Input: part model. Units: mm. Frame: model coordinates. Round coordinates to 2 decimals unless told otherwise and drop trailing zeros. Order: outer loops, then holes, each group sorted by start corner. A loop starts at its lowest first (then second) coordinate and runs counter-clockwise, first axis right, second up. Notation, with made-up numbers: (65, 25) - (84, 25) arc R18 cw to (84, 40) - close; hole circle Ø4 at (-6, -5.75). An arc over 180 degrees is marked (long way). One line per item, written item: value. Start each with the question number.
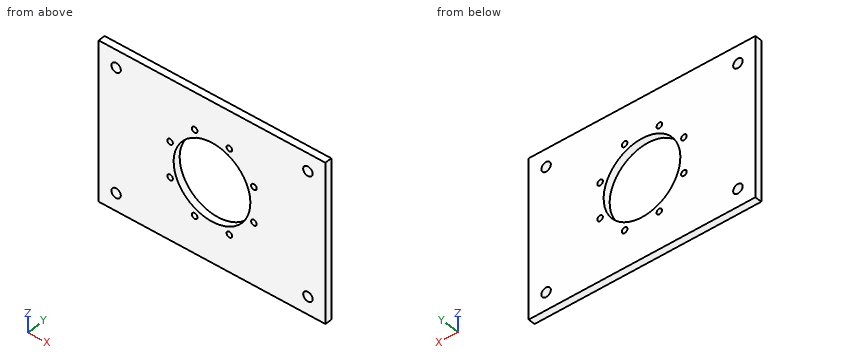
from build123d import *

# Parameters (mm, degrees)
SKETCH1_W           = 325
SKETCH1_H           = 225
SKETCH1_R           = 55
BOSS_EXTRUDE1_DEPTH = 10
SKETCH2_R           = 4
CUT_EXTRUDE1_DEPTH  = 10
CUT_EXTRUDE2_REACH  = 199.895
SKETCH4_R           = 6.75


with BuildPart() as part:
    # Sketch1 → Boss-Extrude1 (new body)
    with BuildSketch(Plane(origin=(0, 0, 0), x_dir=(1, 0, 0), z_dir=(0, 1, 0))):
        Rectangle(SKETCH1_W, SKETCH1_H)
        with Locations(Location((0, 0, 0), (0, 0, 270))):
            Circle(SKETCH1_R, mode=Mode.SUBTRACT)
    extrude(amount=BOSS_EXTRUDE1_DEPTH)

    # Sketch2 → Cut-Extrude1 (cut)
    with BuildSketch(Plane(origin=(0, 0, 0), x_dir=(1, 0, 0), z_dir=(0, 1, 0))):
        with Locations(Location((-24.874423104, -60.052169613, 0), (0, 0, 270))):
            Circle(SKETCH2_R)
        with Locations(Location((-60.052169613, -24.874423104, 0), (0, 0, 270))):
            Circle(SKETCH2_R)
        with Locations(Location((-60.052169613, 24.874423104, 0), (0, 0, 270))):
            Circle(SKETCH2_R)
        with Locations(Location((-24.874423104, 60.052169613, 0), (0, 0, 270))):
            Circle(SKETCH2_R)
        with Locations(Location((24.874423104, 60.052169613, 0), (0, 0, 270))):
            Circle(SKETCH2_R)
        with Locations(Location((60.052169613, 24.874423104, 0), (0, 0, 270))):
            Circle(SKETCH2_R)
        with Locations(Location((60.052169613, -24.874423104, 0), (0, 0, 270))):
            Circle(SKETCH2_R)
        with Locations(Location((24.874423104, -60.052169613, 0), (0, 0, 270))):
            Circle(SKETCH2_R)
    extrude(amount=CUT_EXTRUDE1_DEPTH, mode=Mode.SUBTRACT)

    # Sketch4 → Cut-Extrude2 (cut, up to next)
    with BuildSketch(Plane(origin=(0, 0, 0), x_dir=(1, 0, 0), z_dir=(0, 1, 0)), mode=Mode.PRIVATE) as cut_extrude2_sk1:
        with Locations(Location((137.5, 87.5, 0), (0, 0, 90))):
            Circle(SKETCH4_R)
    cut_extrude2_tool1 = extrude(cut_extrude2_sk1.sketch, amount=CUT_EXTRUDE2_REACH, mode=Mode.PRIVATE) & part.part
    # Sketch4 → Cut-Extrude2 (cut, up to next)
    with BuildSketch(Plane(origin=(0, 0, 0), x_dir=(1, 0, 0), z_dir=(0, 1, 0)), mode=Mode.PRIVATE) as cut_extrude2_sk2:
        with Locations(Location((-137.5, 87.5, 0), (0, 0, 90))):
            Circle(SKETCH4_R)
    cut_extrude2_tool2 = extrude(cut_extrude2_sk2.sketch, amount=CUT_EXTRUDE2_REACH, mode=Mode.PRIVATE) & part.part
    # Sketch4 → Cut-Extrude2 (cut, up to next)
    with BuildSketch(Plane(origin=(0, 0, 0), x_dir=(1, 0, 0), z_dir=(0, 1, 0)), mode=Mode.PRIVATE) as cut_extrude2_sk3:
        with Locations(Location((-137.5, -87.5, 0), (0, 0, 90))):
            Circle(SKETCH4_R)
    cut_extrude2_tool3 = extrude(cut_extrude2_sk3.sketch, amount=CUT_EXTRUDE2_REACH, mode=Mode.PRIVATE) & part.part
    # Sketch4 → Cut-Extrude2 (cut, up to next)
    with BuildSketch(Plane(origin=(0, 0, 0), x_dir=(1, 0, 0), z_dir=(0, 1, 0)), mode=Mode.PRIVATE) as cut_extrude2_sk4:
        with Locations(Location((137.5, -87.5, 0), (0, 0, 90))):
            Circle(SKETCH4_R)
    cut_extrude2_tool4 = extrude(cut_extrude2_sk4.sketch, amount=CUT_EXTRUDE2_REACH, mode=Mode.PRIVATE) & part.part
    add(cut_extrude2_tool1.solids().sort_by_distance((137.5, 0, -87.5))[0], mode=Mode.SUBTRACT)
    add(cut_extrude2_tool2.solids().sort_by_distance((-137.5, 0, -87.5))[0], mode=Mode.SUBTRACT)
    add(cut_extrude2_tool3.solids().sort_by_distance((-137.5, 0, 87.5))[0], mode=Mode.SUBTRACT)
    add(cut_extrude2_tool4.solids().sort_by_distance((137.5, 0, 87.5))[0], mode=Mode.SUBTRACT)


solid = part.part
1. Section C-C (x = -137.5). Return the cut outline in (y, z), then the cut area to 3 significant figures.
2. Section A-A (x = -49). Return the cut outline in (y, z), then the cut area to 3 significant figures.
3. Line query: line 1 (X direction, y = 6, z = -87.5); line 2 (Z direction, x = -137.5, y = 3.5); line 3 (X direction, y = 1, z = 85). Output: solid intervals per line, ascending. Write a range as from..to.
4. Section D-D (z = 84.5). Return the cut outline in (x, y), then the cut area to 3 significant figures.
5. Section B-B (z = 49). Return the cut outline in (x, y), then the cut area to 3 significant figures.
Solved:
1. outline: (0, -112.5) - (10, -112.5) - (10, -94.25) - (0, -94.25) - close; (0, -80.75) - (10, -80.75) - (10, 80.75) - (0, 80.75) - close; (0, 94.25) - (10, 94.25) - (10, 112.5) - (0, 112.5) - close
1. area: 1,980 mm²
2. outline: (0, -112.5) - (10, -112.5) - (10, -24.98) - (0, -24.98) - close; (0, 24.98) - (10, 24.98) - (10, 112.5) - (0, 112.5) - close
2. area: 1,750 mm²
3. line 1: x = -162.5..-144.25, -130.75..130.75, 144.25..162.5
3. line 2: z = -112.5..-94.25, -80.75..80.75, 94.25..112.5
3. line 3: x = -162.5..-143.77, -131.23..131.23, 143.77..162.5
4. outline: (-162.5, 0) - (-143.55, 0) - (-143.55, 10) - (-162.5, 10) - close; (-131.45, 0) - (131.45, 0) - (131.45, 10) - (-131.45, 10) - close; (143.55, 0) - (162.5, 0) - (162.5, 10) - (143.55, 10) - close
4. area: 3,010 mm²
5. outline: (-162.5, 0) - (-24.98, 0) - (-24.98, 10) - (-162.5, 10) - close; (24.98, 0) - (162.5, 0) - (162.5, 10) - (24.98, 10) - close
5. area: 2,750 mm²
